```python
from build123d import *

# Parameters (mm, degrees)
F0_W     = 203.2
F0_H     = 101.6
F1_DEPTH = 101.6
F2_W     = 101.6
F2_H     = 76.2
F3_DEPTH = 50.8
F5_DEPTH = 50.8
F7_DEPTH = 203.201


with BuildPart() as f1:
    # F0 (on Front) → F1 (new body)
    with BuildSketch(Plane.XZ):
        with Locations((-7.6962560415, -14.9830856085)):
            Rectangle(F0_W, F0_H)
    extrude(amount=F1_DEPTH)

    # F2 (on face) → F3 (cut)
    with BuildSketch(Plane.XZ.offset(101.6)):
        with Locations((-7.826578486, -2.2830856085)):
            Rectangle(F2_W, F2_H)
    extrude(amount=-F3_DEPTH, mode=Mode.SUBTRACT)

    # F4 (on face) → F5 (cut)
    with BuildSketch(Plane(origin=(-109.2962560415, 0, 0), x_dir=(0, -1, 0), z_dir=(-1, 0, 0))):
        Polygon((50.8, 35.8169143915), (101.6, -40.3830856085), (101.6, 35.8169143915), align=None)
    extrude(amount=-F5_DEPTH, mode=Mode.SUBTRACT)

    # F6 (on face) → F7 (cut, through all)
    with BuildSketch(Plane.YZ.offset(93.9037439585)):
        Polygon((-101.6, 35.8169143915), (-101.6, -40.4823369622), (-50.8, 35.8169143915), align=None)
    extrude(amount=-F7_DEPTH, mode=Mode.SUBTRACT)


solid = f1.part
```
Geometry: final body of the model. Coordinates: model frame, mm. A direction names the side the tool comes from. Round coordinates to 2 decimals unless told otherwise and drop trailing zeros. Write each loop counter-clockwise with the first axis right and the second up, starting at its lowest first coordinate (ties: lowest second). Pieces come first, ordered by that corner, then holes.
Item 1: Section query D-D (x = -76). Return loops of the section in (y, z).
Item 2: Section query B-B (z = -24). Return loops of the section in (x, y), plus the area to 3 significant figures.
Item 3: Pin query (flat end, axial travel): P1, Ø23, axis at x = -23, z = -1.5, coming from the -Y side; P2, Ø2, axis at x = 3, y = -89, coming from the +Z side. Return the tip coordinate at first contact, or that it passes through.
Item 4: Section query C-C (z = 13). Return loops of the section in (x, y), plus the area to 3 significant figures.
Item 5: Set-up query: faces 1 (the face through (61.46, -76.56, -2.87)), 2 (the face through (-9, -77, -40.383)). Return all of +Z, -Z, +X, -X, +Y, -Y with unobstructed straight access to the full face (end or side cutting, diameter ignored); none if empty.
Item 6: Section query A-A (x = -54.5). Return loops of the section in (y, z), plus the area to 3 significant figures.
Item 7: Material intervals for L1, parallel to X at y = -59.5, z = -16.5; L2, parallel to Y at x = -48.5, z = -24; L3, parallel to Z at x = 39, y = -85.5, sorted ascending.
Completed:
1. outline: (-101.6, -65.78) - (0, -65.78) - (0, 35.82) - (-50.8, 35.82) - (-101.6, -40.48) - close
2. outline: (-109.3, -90.63) - (-58.63, -90.63) - (-58.63, -50.8) - (42.97, -50.8) - (42.97, -90.63) - (93.9, -90.63) - (93.9, 0) - (-109.3, 0) - close
2. area: 14,400 mm2
3. P1: stops at y = -50.8
3. P2: stops at z = -40.38
4. outline: (-109.3, -65.99) - (-58.63, -65.99) - (-58.63, -50.8) - (42.97, -50.8) - (42.97, -65.99) - (93.9, -65.99) - (93.9, 0) - (-109.3, 0) - close
4. area: 11,900 mm2
5. face 1: +Z, +X, -X, -Y
5. face 2: +Z, -Y
6. outline: (-101.6, -65.78) - (0, -65.78) - (0, 35.82) - (-50.8, 35.82) - (-50.8, -40.38) - (-101.53, -40.38) - (-101.6, -40.48) - close
6. area: 6,450 mm2
7. L1: x = -109.3 to -58.63, 42.97 to 93.9
7. L2: y = -50.8 to 0
7. L3: z = -65.78 to -40.38
